Could you check a few things on this model? Use its own coordinates, in mm. A direction names the side the tool comes from. Round coordinates to 2 decimals unless told otherwise and drop trailing zeros. Loops run counter-clockwise (first coordinate to the right, second up) from the corner with the lowest first, then second, coordinate; pieces in that order, holes last. Notation, with made-up numbers: M -24,-5.75 L -13,-5.75 A35 ccw -13,33.25 Z; hole C 73.5,55.25 d11. An arc over 180 degrees is marked long. One line per item, written item: value. Start each with the question number.
Q1. Imagine slicing it at B-B (y = 140). Please give me the cut outline in (x, z).
Q2. Imagine slicing it at A-A (y = 35). Please give me the cut outline in (x, z), then the cut area to 3 significant figures.
Q3. Which directions (+Z, -Z, +X, -X, +Y, -Y) give clear straight access to the entire face, cutting with the end or side of a thin tool? Please do faces 1 (the face through (-3, 203, 29.962)), 2 (the face through (-2, 32, 14.087)), 3 (the face through (9, 6.35, 6)).
Q4. Please list where these lines run through material, in increasing order: line 1 along X through (y, z) = (18, 14.5); line 2 along Y through (x, z) = (7, 10); line 3 along Z through (x, y) = (-16, 176.5).
Q5. Thinking about a two-plate mould opening in X: for faces 4 (the face through (-7.972, 32, 22)), 5 (the face through (9, 57.15, 6)), 6 (the face through (0.769, 31, 6)), which applies, released by +X, released by -X, zero draft, split by the parting line, or undercut?
from build123d import *

# Parameters (mm, degrees)
F0_W     = 38.1
F0_H     = 50.8
F1_DEPTH = 412.75
F3_DEPTH = 15.875
F5_DEPTH = 15.875
F6_R     = 6.35


with BuildPart() as f1:
    # F0 (on Front) → F1 (new body)
    with BuildSketch(Plane.XZ):
        with Locations((-2.406317, 4.562353)):
            Rectangle(F0_W, F0_H)
    extrude(amount=-F1_DEPTH)

    # F2 (on face) → F3 (cut)
    with BuildSketch(Plane.YZ.offset(16.643683)):
        with BuildLine():
            Line((53.975, 12.7), (9.525, 12.7))
            ThreePointArc((9.525, 12.7), (7.279936, 11.770064), (6.35, 9.525))
            Line((6.35, 9.525), (6.35, 3.175))
            ThreePointArc((6.35, 3.175), (7.279936, 0.929936), (9.525, 0))
            Line((9.525, 0), (53.975, 0))
            ThreePointArc((53.975, 0), (56.220064, 0.929936), (57.15, 3.175))
            Line((57.15, 3.175), (57.15, 9.525))
            ThreePointArc((57.15, 9.525), (56.220064, 11.770064), (53.975, 12.7))
        make_face()
    extrude(amount=-F3_DEPTH, mode=Mode.SUBTRACT)

    # F4 (on face) → F5 (cut)
    with BuildSketch(Plane.XY.offset(29.962353)):
        with BuildLine():
            ThreePointArc((-4.797424, 57.15), (-7.042488, 56.220064), (-7.972424, 53.975))
            Line((-7.972424, 53.975), (-7.972424, 9.525))
            ThreePointArc((-7.972424, 9.525), (-7.042488, 7.279936), (-4.797424, 6.35))
            Line((-4.797424, 6.35), (1.552576, 6.35))
            ThreePointArc((1.552576, 6.35), (3.79764, 7.279936), (4.727576, 9.525))
            Line((4.727576, 9.525), (4.727576, 53.975))
            ThreePointArc((4.727576, 53.975), (3.79764, 56.220064), (1.552576, 57.15))
            Line((1.552576, 57.15), (-4.797424, 57.15))
        make_face()
    extrude(amount=-F5_DEPTH, mode=Mode.SUBTRACT)

    # F6
    f6_edges = [f1.edges().sort_by_distance(p)[0] for p in [
        (16.643683, 206.375, -20.837647),
        (-21.456317, 206.375, -20.837647),
        (16.643683, 206.375, 29.962353),
        (-21.456317, 206.375, 29.962353),
    ]]
    fillet(f6_edges, radius=F6_R)


solid = f1.part
Report:
1. outline: M -21.46,-14.49 A6.35 ccw -15.11,-20.84 L 10.29,-20.84 A6.35 ccw 16.64,-14.49 L 16.64,23.61 A6.35 ccw 10.29,29.96 L -15.11,29.96 A6.35 ccw -21.46,23.61 Z
2. outline: M -21.46,-14.49 A6.35 ccw -15.11,-20.84 L 10.29,-20.84 A6.35 ccw 16.64,-14.49 L 16.64,0 L 0.77,0 L 0.77,12.7 L 16.64,12.7 L 16.64,23.61 A6.35 ccw 10.29,29.96 L 4.73,29.96 L 4.73,14.09 L -7.97,14.09 L -7.97,29.96 L -15.11,29.96 A6.35 ccw -21.46,23.61 Z
2. area: 1,500 mm²
3. face 1: +Z, +X, -X, +Y, -Y
3. face 2: +Z
3. face 3: +X
4. line 1: x = -21.46 to -7.97, 4.73 to 16.64
4. line 2: y = 0 to 6.39, 57.11 to 412.75
4. line 3: z = -20.77 to 29.9
5. face 4: undercut
5. face 5: zero draft
5. face 6: released by +X
